Autodesk Inventor part; units mm, degrees
ref_plane "Arbeitsebene1" through (0, 0, 39.5) normal (0, 0, 1) x (1, 0, 0)
ref_plane "Arbeitsebene2" through (-4, 50, 0) normal (0, 1, 0) x (1, 0, 0)
ref_plane "Arbeitsebene3" through (-4, 20, 0) normal (0, -1, 0) x (1, 0, 0)
sketch "Skizze1" plane through (0, 0, 0) normal (0, 0, 1) x (1, 0, 0)
  circle A0 centre (-17, 35) radius 12.5
  line L0 (0, 70) -> (0, 0)
  circle A1 centre (-17, 26.5) radius 1.6
  circle A2 centre (-17, 43.5) radius 1.6
  circle A3 centre (-17, 35) radius 5.5
  line L1 (3, 0) -> (0, 0)
  line L2 (0, 70) -> (-4, 70)
  line L3 (-4, 70) -> (-4, 0)
  line L4 (-4, 0) -> (0, 0)
  line L5 (0, 0) -> (0, 70)
  line L6 (-26.5845, 43.0242) -> (-4, 70)
  line L7 (-26.5845, 26.9758) -> (-4, 0)
  line L8 (0, 0) -> (-41.7952, 0)
  line L9 (-41.7952, 0) -> (-41.7952, 70)
  line L10 (-41.7952, 70) -> (0, 70)
  line L11 (0, 70) -> (0, 0)
  point P0 (0, 0)
  point P1 (0, 55)
  dimension "d0" = 25
  dimension "d2" = 8.5
  dimension "d3" = 17
  dimension "d6" = 3.2
  dimension "d7" = 3.2
  dimension "d8" = 11
  dimension "d10" = 70
  dimension "d11" = 17
  dimension "d23" = 4
extrude "Extrusion1" add sketch "Skizze1" along normal blind 7 contours A0 | A0 L6 L3 L7
ref_plane "Arbeitsebene1" through (0, 0, 39.5) normal (0, 0, 1) x (1, 0, 0)
extrude "Extrusion8" add sketch "Skizze1" along normal blind 15 contours L2 L0 L4 L3
ref_plane "Arbeitsebene2" through (-4, 50, 0) normal (0, 1, 0) x (1, 0, 0)
ref_plane "Arbeitsebene3" through (-4, 20, 0) normal (0, -1, 0) x (1, 0, 0)
sketch "Skizze8" plane through (-4, 50, 0) normal (0, 1, 0) x (1, 0, 0)
  line L0 (0, -15) -> (4, -15)
  line L1 (0, -15) -> (-15.5, -7)
  line L2 (-15.5, -7) -> (0, -7)
  line L3 (0, -7) -> (0, -15)
  line L4 (0, -7) -> (-22.5845, -7)
  point P0 (4, 0)
  dimension "d59" = 15.5
sketch "Skizze9" plane through (-4, 20, 0) normal (0, -1, 0) x (1, 0, 0)
  line L0 (0, 15) -> (-15.5, 7)
  line L1 (0, 7) -> (0, 15)
  line L2 (-15.5, 7) -> (0, 7)
  line L3 (-15.5, 7) -> (0, 15)
  line L4 (-22.5845, 7) -> (0, 7)
  line L5 (0, 7) -> (0, 15)
  line L6 (-15.5, 7) -> (0, 7)
  point P0 (4, 0)
extrude "Extrusion9" add sketch "Skizze9" along normal blind 5
extrude "Extrusion10" add sketch "Skizze8" along normal blind 5
extrude "Extrusion11" cut sketch "Skizze1" along normal blind 20 contours A0 L7 L8 L9 L10 L6
sketch "Skizze10" plane through (-4, 0, 7) normal (-1, 0, 0) x (0, 0, 1)
  circle A0 centre (4, 7.5) radius 2
  circle A1 centre (4, 62.5) radius 2
  line L0 (0, 70) -> (8, 70)
  line L1 (1.5184, 55) -> (8, 55)
  line L2 (0, 0) -> (8, 0)
  line L3 (8, 15) -> (8, 0)
  line L4 (8, 70) -> (8, 55)
  line L5 (-7, 26.9758) -> (-7, 0)
  dimension "d67" = 4
  dimension "d68" = 4
  dimension "d69" = 7.5
  dimension "d71" = 7.5
  dimension "d72" = 4
  dimension "d73" = 4
  dimension "d76" = 11
extrude "Extrusion12" cut sketch "Skizze10" against normal blind 4
chamfer "Fase1" distance 2 angle 45 2 edges at (-18.6, 43.5, 0) (-18.6, 26.5, 0)
equation "\"d6\" = d7"
equation "\"d68\" = d67"
equation "\"d71\" = d69"
properties part number "motor mount"
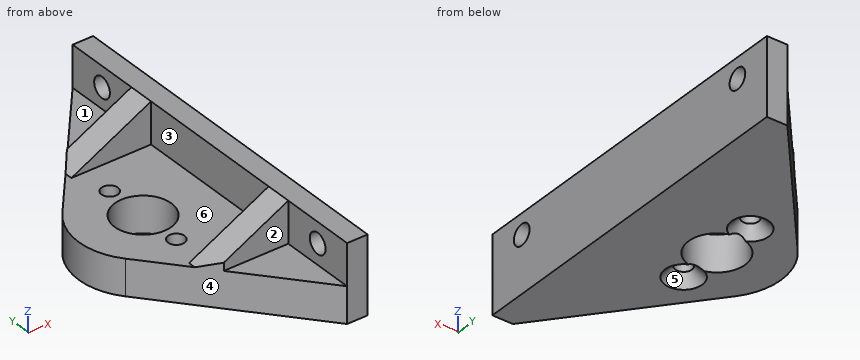
Source: CAD feature listing. Evaluate the final solid. Frame: model axes, mm. Face numbers are marked on the shaded views. A direction names the side the tool comes from. Coordinates: 2 decimals unless noted, no trailing zeros. Loops run counter-clockwise (first coordinate to the right, second up) from the corner with the lowest first, then second, coordinate; pieces in that order, holes last. Notation, with made-up numbers: (-12, 0) -> (20, 0) arc R28 cw to (20, 27) -> close; hole circle Ø5 at (63, -15). An arc over 180 degrees is marked (long way). Answer in a Markdown table with one row per item. Add a question column.
Q1. Section C-C on x = -9.5. Return the cut outline in (y, z).
Q2. Ray query, line 1 along Y through (x, z) = (-1.65, 11); line 2 along Y through (x, z) = (-17, 3.65); line 3 along X through (y, z) = (34, 13). Return the intervals inside material, ascending.
Q3. Section A-A on z = 11. Return the cut outline in (x, y).
Q4. Section B-B on y = 7.5. Return the cut outline in (x, z).
Q5. Pull-direction query (X, two-part tool) for the marked faces 4, 5 and 6; classes: pulls with the +X half, pulls with the -X half, needs draft (parallel to the pull), parting line crosses it, or undercut.
Q6. Section D-D on z = 5.5. Return the cut outline in (x, y), and give its area (3 significant figures).
Q7. Reachability of the marked faces 1, 2 and 3 from +Z, -Z, +X, -X, +Y, -Y: full face, straight path, thin tool, end or side. Return the list, or none.
Q8. Contact query for flat-ended pins moving along their axis: pin 1 Ø3 at (x, y) = (-17, 43.5) entering from +Z; pin 2 Ø6.5 at (y, z) = (33, 12) entering from -X; pin 3 Ø6.5 at (x, z) = (-10, 9.5) entering from +Y; pin 4 Ø9 at (y, z) = (62.5, 9.5) entering from -X. Output: stop coordinate, or through.
Computed values:
| question | item | result |
|---|---|---|
| 1 | outline | (6.57, 0) -> (63.43, 0) -> (63.43, 7) -> (55, 7) -> (55, 12.16) -> (50, 12.16) -> (50, 7) -> (20, 7) -> (20, 12.16) -> (15, 12.16) -> (15, 7) -> (6.57, 7) -> close |
| 2 | line 1 | y = 0 to 5.5, 9.5 to 60.5, 64.5 to 70 |
| 2 | line 2 | y = 15.53 to 24.9, 28.1 to 29.5, 40.5 to 41.9, 45.1 to 54.47 |
| 2 | line 3 | x = -4 to 0 |
| 3 | outline | (-11.75, 15) -> (-4, 15) -> (-4, 9.5) -> (0, 9.5) -> (0, 60.5) -> (-4, 60.5) -> (-4, 55) -> (-11.75, 55) -> (-11.75, 50) -> (-4, 50) -> (-4, 20) -> (-11.75, 20) -> close; (-4, 0) -> (0, 0) -> (0, 5.5) -> (-4, 5.5) -> close; (-4, 64.5) -> (0, 64.5) -> (0, 70) -> (-4, 70) -> close |
| 4 | outline | (-10.28, 0) -> (0, 0) -> (0, 9) -> (-4, 9) -> (-4, 7) -> (-10.28, 7) -> close; (-4, 13) -> (0, 13) -> (0, 15) -> (-4, 15) -> close |
| 5 | face 4 | pulls with the -X half |
| 5 | face 5 | undercut |
| 5 | face 6 | needs draft |
| 6 | outline | (-26.58, 26.98) -> (-4, 0) -> (0, 0) -> (0, 70) -> (-4, 70) -> (-26.58, 43.02) arc R12.5 ccw to start; hole circle Ø11 at (-17, 35); hole circle Ø3.2 at (-17, 26.5); hole circle Ø3.2 at (-17, 43.5) |
| 6 | area | 1,170 mm^2 |
| 7 | face 1 | +Z, -X, +Y |
| 7 | face 2 | +Z, -X, -Y |
| 7 | face 3 | +Z, -X |
| 8 | pin 1 | passes through |
| 8 | pin 2 | stops at x = -4 |
| 8 | pin 3 | stops at y = 65.31 |
| 8 | pin 4 | stops at x = -13.41 |
